Check sheet for the modelled part. Datum: model origin and axes. Units: mm. A direction names the side the tool comes from. Coordinates: 2 decimals unless noted, no trailing zeros. Loops run counter-clockwise (first coordinate to the right, second up) from the corner with the lowest first, then second, coordinate; pieces in that order, holes last. Notation, with made-up numbers: (7, -15) - (26, -15) arc R26 ccw to (26, 23) - close; hole circle Ø2 at (75.5, 86.25). An arc over 180 degrees is marked (long way). Write each question's results on one line, items separated by ' | '. Start each with the question number.
1. Tool access check on faces 4 (the face through (-158, 148, -24)), 5 (the face through (-158, 156.25, -45)), 6 (the face through (-162, 129.25, 86)). Record the directions out of +Z, -Z, +X, -X, +Y, -Y that give a thin tool (end or side, any length) a straight path to the whole face; none if there is none.
2. Cross-section at B-B (y = 86). Record the cut outline in (x, z).
3. Thickness scan on line 1 (Z direction, x = -165, y = 156.75); line 2 (Z direction, x = -158, y = 141); line 3 (X direction, y = 156.75, z = -46.5). Record the ranges inside material, lowest first. Write a range as [from, to].
4. Cross-section at A-A (z = -46.5). Record the cut outline in (x, y).
5. Gauge pin test, flat ends, axial feed: P1, Ø12.5, axis at x = -160.5, z = 91, coming from the -Y side; P2, Ø8, axis at x = -164, y = 102.5, coming from the +Z side; P3, Ø1.5, axis at x = -149, z = -25, coming from the +Y side. Record the tip position at first contact, or that the pin passes through.
6. Cross-section at D-D (y = 116). Record the cut outline in (x, z).
7. Draft check along X on faces 1 (the face through (-151, 157, 89)), 2 (the face through (-167.5, 114, 85)), 3 (the face through (-158, 156.25, 89)). Enter one of: released by +X, released by -X, zero draft, split by the parting line, or undercut.
8. Cross-section at C-C (z = 51.5). Record the cut outline in (x, y), and give its area (3 significant figures).
```python
from build123d import *

# Parameters (mm, degrees)
CYLINDER030_R             = 1.5
CYLINDER030_DEPTH         = 10
CYLINDER031_R             = 1.5
CYLINDER031_DEPTH         = 10
CYLINDER032_R             = 1.5
CYLINDER032_DEPTH         = 10
CYLINDER029_R             = 1.5
CYLINDER029_DEPTH         = 10
CYLINDER028_R             = 3
CYLINDER028_DEPTH         = 10
CYLINDER027_R             = 3
CYLINDER027_DEPTH         = 10
BOX036_W                  = 30
BOX036_H                  = 9
BOX036_DEPTH              = 11
BOX037_W                  = 1
BOX037_H                  = 25.5
BOX037_DEPTH              = 23.2
BOX038_W                  = 1
BOX038_H                  = 25.5
BOX038_DEPTH              = 23.2
BOX002_W                  = 17
BOX002_H                  = 16.5
BOX002_DEPTH              = 13.25
BOX035_W                  = 17
BOX035_H                  = 65
BOX035_DEPTH              = 13.25
BOX034_W                  = 89
BOX034_H                  = 118
BOX034_DEPTH              = 28
FILLET022_R               = 2
FILLET022_ROLL_ANGLE      = -90
FILLET022_PLACEMENT_ANGLE = 90


with BuildPart() as cylinder030:
    # Cylinder030 → Cylinder030 (new body)
    with BuildSketch(Plane(origin=(85, -9.5, 20.25), x_dir=(0, 0, -1), z_dir=(1, 0, 0))):
        Circle(CYLINDER030_R)
    extrude(amount=CYLINDER030_DEPTH)


with BuildPart() as cylinder031:
    # Cylinder031 → Cylinder031 (new body)
    with BuildSketch(Plane(origin=(85, 127.5, 6.25), x_dir=(0, 0, -1), z_dir=(1, 0, 0))):
        Circle(CYLINDER031_R)
    extrude(amount=CYLINDER031_DEPTH)


with BuildPart() as cylinder032:
    # Cylinder032 → Cylinder032 (new body)
    with BuildSketch(Plane(origin=(85, 127.5, 20.25), x_dir=(0, 0, -1), z_dir=(1, 0, 0))):
        Circle(CYLINDER032_R)
    extrude(amount=CYLINDER032_DEPTH)


with BuildPart() as mount_small_cyl:
    # Cylinder029 → Cylinder029 (new body)
    with BuildSketch(Plane(origin=(85, -9.5, 6.25), x_dir=(0, 0, -1), z_dir=(1, 0, 0))):
        Circle(CYLINDER029_R)
    extrude(amount=CYLINDER029_DEPTH)

    # Fusion021: union Cylinder030, Cylinder031, Cylinder032
    add(cylinder030.part)
    add(cylinder031.part)
    add(cylinder032.part)


with BuildPart() as cylinder028:
    # Cylinder028 → Cylinder028 (new body)
    with BuildSketch(Plane(origin=(93, 121, 4.5), x_dir=(0, 0, 1), z_dir=(-1, 0, 0))):
        Circle(CYLINDER028_R)
    extrude(amount=CYLINDER028_DEPTH)


with BuildPart() as mount_cyl:
    # Cylinder027 → Cylinder027 (new body)
    with BuildSketch(Plane(origin=(93, -3, 4.5), x_dir=(0, 0, 1), z_dir=(-1, 0, 0))):
        Circle(CYLINDER027_R)
    extrude(amount=CYLINDER027_DEPTH)

    # Fusion020: union Cylinder028
    add(cylinder028.part)


with BuildPart() as mount_cyl_1:
    # Fusion020 placement: moved
    add(mount_cyl.part.moved(Location((0, 0, 9.25))))


with BuildPart() as power:
    # Box036 → Box036 (new body)
    with BuildSketch(Plane(origin=(32, -9, 11.75), x_dir=(1, 0, 0), z_dir=(0, 0, 1))):
        with Locations((15, 4.5)):
            Rectangle(BOX036_W, BOX036_H)
    extrude(amount=BOX036_DEPTH)


with BuildPart() as mount1:
    # Box037 → Box037 (new body)
    with BuildSketch(Plane(origin=(89, -15.5, 2.25), x_dir=(1, 0, 0), z_dir=(0, 0, 1))):
        with Locations((0.5, 12.75)):
            Rectangle(BOX037_W, BOX037_H)
    extrude(amount=BOX037_DEPTH)


with BuildPart() as mount2:
    # Box038 → Box038 (new body)
    with BuildSketch(Plane(origin=(89, 108, 2.25), x_dir=(1, 0, 0), z_dir=(0, 0, 1))):
        with Locations((0.5, 12.75)):
            Rectangle(BOX038_W, BOX038_H)
    extrude(amount=BOX038_DEPTH)


with BuildPart() as cube020:
    # Box002 → Box002 (new body)
    with BuildSketch(Plane(origin=(72, 88.5, 7), x_dir=(1, 0, 0), z_dir=(0, 0, 1))):
        with Locations((8.5, 8.25)):
            Rectangle(BOX002_W, BOX002_H)
    extrude(amount=BOX002_DEPTH)


with BuildPart() as cube019:
    # Box035 → Box035 (new body)
    with BuildSketch(Plane(origin=(72, 14.25, 7), x_dir=(1, 0, 0), z_dir=(0, 0, 1))):
        with Locations((8.5, 32.5)):
            Rectangle(BOX035_W, BOX035_H)
    extrude(amount=BOX035_DEPTH)


with BuildPart() as switch:
    # Box034 → Box034 (new body)
    with BuildSketch(Plane.XY):
        with Locations((44.5, 59)):
            Rectangle(BOX034_W, BOX034_H)
    extrude(amount=BOX034_DEPTH)

    # Cut023: cut Cube019
    add(cube019.part, mode=Mode.SUBTRACT)

    # Cut024: cut Cube020
    add(cube020.part, mode=Mode.SUBTRACT)

    # Fusion019: union Power, mount1, mount2
    add(power.part)
    add(mount1.part)
    add(mount2.part)

    # Cut025: cut mount_cyl
    add(mount_cyl_1.part, mode=Mode.SUBTRACT)

    # Cut026: cut mount_small_cyl
    add(mount_small_cyl.part, mode=Mode.SUBTRACT)

    # Fillet022
    fillet022_edges = [switch.edges().sort_by_distance(p)[0] for p in [
        (44.5, 0, 0),
        (44.5, 0, 28),
        (0, 59, 0),
        (44.5, 118, 0),
        (89, 59, 0),
        (89, 59, 28),
        (0, 59, 28),
    ]]
    fillet(fillet022_edges, radius=FILLET022_R)


with BuildPart() as switch_1:
    # Fillet022 roll: moved
    add(switch.part.rotate(Axis((0, 0, 0), (1, 0, 0)), FILLET022_ROLL_ANGLE))


with BuildPart() as switch_2:
    # Fillet022 placement: moved
    add(switch_1.part.moved(Location((-144.75, 67.25, 81))).rotate(Axis((-144.75, 67.25, 81), (0, 0, 1)), FILLET022_PLACEMENT_ANGLE))


solid = switch_2.part
```
Established:
1) face 4: +Y | face 5: -Z, +X, -X, -Y | face 6: +Z, +X, -X
2) outline: (-172.75, -37) - (-146.75, -37) arc R2 ccw to (-144.75, -35) - (-144.75, 79) arc R2 ccw to (-146.75, 81) - (-170.75, 81) arc R2 ccw to (-172.75, 79) - close
3) line 1: [-52.5, -48], [-45, -27], [71, 89], [92, 96.5] | line 2: [-37, -24], [-7.5, 1.75], [66.75, 81] | line 3: [-170.2, -166.5], [-163.5, -152.5], [-149.5, -147]
4) outline: (-170.2, 156.25) - (-166.5, 156.25) - (-166.5, 157.25) - (-170.2, 157.25) - close; (-163.5, 156.25) - (-152.5, 156.25) - (-152.5, 157.25) - (-163.5, 157.25) - close; (-149.5, 156.25) - (-147, 156.25) - (-147, 157.25) - (-149.5, 157.25) - close
5) P1: y = 99.25 | P2: z = 90 | P3: y = 156.25
6) outline: (-172.75, -37) - (-146.75, -37) arc R2 ccw to (-144.75, -35) - (-144.75, 79) arc R2 ccw to (-146.75, 81) - (-156.5, 81) - (-156.5, 90) - (-167.5, 90) - (-167.5, 81) - (-170.75, 81) arc R2 ccw to (-172.75, 79) - close
7) face 1: undercut | face 2: released by -X | face 3: zero draft
8) outline: (-172.75, 69.25) arc R2 ccw to (-170.75, 67.25) - (-146.75, 67.25) arc R2 ccw to (-144.75, 69.25) - (-144.75, 154.25) arc R2 ccw to (-146.75, 156.25) - (-151.75, 156.25) - (-151.75, 139.25) - (-165, 139.25) - (-165, 156.25) - (-170.75, 156.25) arc R2 ccw to (-172.75, 154.25) - close | area: 2,260 mm^2
